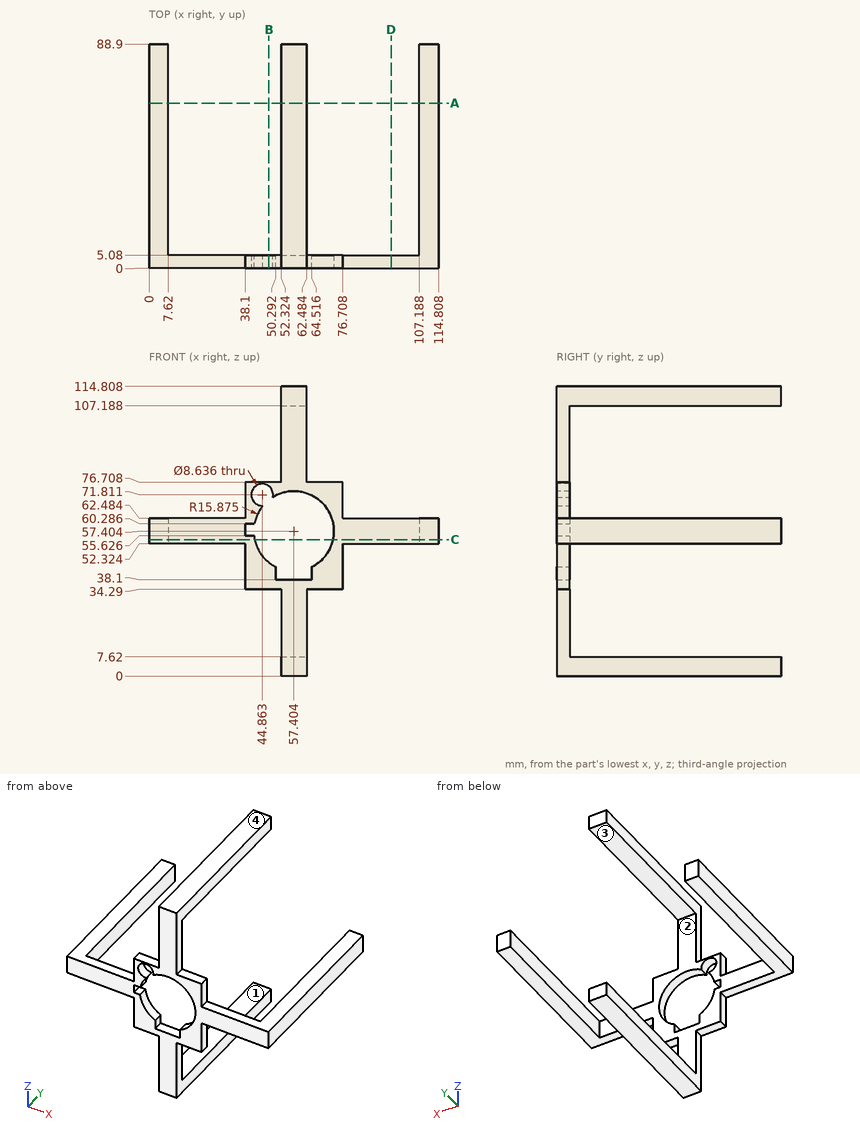
Job drawing, mm, ordinate dimensions from the low corner. One solid piece. A direction names the side the tool comes from. Round coordinates to 2 decimals unless told otherwise and drop trailing zeros. Write each loop counter-clockwise with the first axis right and the second up, starting at its lowest first coordinate (ties: lowest second). Pieces come first, ordered by that corner, then holes.
1) Drill centre lines: probe 1 along X at (y, z) = (51, 60); probe 2 along Y at (x, z) = (56.5, 19.5). Where is each one in solid material? Low to high.
2) Band-saw the part on A-A, the plane y = 65.5. List the corners of the cut face in (x, z), and give its area (3 significant figures).
3) Band-saw the part on C-C, the plane z = 54. List the corners of the cut face in (x, y), and give its area (3 significant figures).
4) 3-axis set-ups, long thin cutter, end or side, ignore diameter. For the marked faces 3 and 4: which of +Z, -Z, +X, -X, +Y, -Y reach the whole face in a straight line?
5) Band-saw the part on D-D, the plane x = 96. List the corners of the cut face in (y, z), and give its area (3 significant figures).
6) Pin check, flat tips, straight feed: pin 1 (4 mm diameter, centred on y = 2, z = 40.5, fed in from -X); pin 2 (4 mm diameter, centred on y = 3, z = 39, fed in from +X); pin 3 (1.1 mm diameter, centred on x = 40.5, y = 2.5, fed in from +Z). Stop position of each tip, or through.
7) Band-saw the part on B-B, the plane x = 47.5. List the corners of the cut face in (y, z).
8) Mould opens along X. For the marked faces 1 and 2 say: +X half, -X half, draft (parallel to the pull), parting line (faces both ways), or undercut.
Ans:
1. probe 1: x = 0 to 7.62, 107.19 to 114.81
1. probe 2: y = 0 to 5.08
2. outline: (0, 52.32) - (7.62, 52.32) - (7.62, 62.48) - (0, 62.48) - close; (52.32, 0) - (62.48, 0) - (62.48, 7.62) - (52.32, 7.62) - close; (52.32, 107.19) - (62.48, 107.19) - (62.48, 114.81) - (52.32, 114.81) - close; (107.19, 52.32) - (114.81, 52.32) - (114.81, 62.48) - (107.19, 62.48) - close
2. area: 310 mm2
3. outline: (0, 0) - (41.9, 0) - (41.9, 5.08) - (7.62, 5.08) - (7.62, 88.9) - (0, 88.9) - close; (72.91, 0) - (114.81, 0) - (114.81, 88.9) - (107.19, 88.9) - (107.19, 5.08) - (72.91, 5.08) - close
3. area: 1,700 mm2
4. face 3: +X, -X, +Y
4. face 4: +Z, +X, -X, +Y, -Y
5. outline: (0, 52.32) - (5.08, 52.32) - (5.08, 62.48) - (0, 62.48) - close
5. area: 51.6 mm2
6. pin 1: stops at x = 38.1
6. pin 2: stops at x = 76.71
6. pin 3: stops at z = 76.71
7. outline: (0, 34.29) - (5.08, 34.29) - (5.08, 45) - (0, 45) - close; (0, 75.23) - (5.08, 75.23) - (5.08, 76.71) - (0, 76.71) - close
8. face 1: draft
8. face 2: undercut
